Design review of the part shown in the three views and the two pictorial views. Dimensions are in mm from the part's minimum x, y and z. A direction names the side the tool comes from. Coordinates: 2 decimals unless noted, no trailing zeros. Write each loop counter-clockwise with the first axis right and the second up, starting at its lowest first coordinate (ties: lowest second). Pieces come first, ordered by that corner, then holes. Notation, with made-up numbers: (79, 19) -> (123, 19) arc R29 ccw to (123, 51) -> close; hole circle Ø9 at (1.5, -34). An arc over 180 degrees is marked (long way). Answer in a Markdown table with one row per item. Add a question column.
Item 1: Take a section at D-D, the plane y = 31. Write out the cut boundary in (x, z).
Item 2: Draft analysis for pull direction X (two halves, no side actions). For the marked faces 3 and 4, state which applies: released by +X, released by -X, zero draft, split by the parting line, or undercut.
Item 3: Take a section at B-B, the plane x = 45.5. Write out the cut boundary in (y, z).
Item 4: Clearance check with flat-ended pins moving along their axes: P1, Ø6, axis at x = 34.5, z = 41.5, coming from the +Y side; P2, Ø3.5, axis at x = 63, y = 1.5, coming from the -Z side; P3, Ø0.9, axis at x = 65.5, y = 1, coming from the +Z side; P4, Ø12, axis at x = 29, z = 6.5, coming from the -Y side. State where each tip first meets the part, or that it passes through.
Item 5: Take a section at C-C, the plane x = 63.5. Write out the cut boundary in (y, z), and give its area (3 significant figures).
Item 6: To check wall thickness, follow line 1 (X direction, y = 1, z = 24); line 2 (X direction, y = 10, z = 14.5); line 3 (Z direction, x = 63.5, y = 1.7). State the ranges of each line that lie inside material, in increasing order.
Item 7: For the marked faces 1 and 2, list the 3-axis set-ups (+Z, -Z, +X, -X, +Y, -Y) from which the entire face can be reached by the end or side of a thin tool; tool diameter is ignored.
Item 8: Take a section at A-A, the plane z = 24.25. Write out the cut boundary in (x, y).
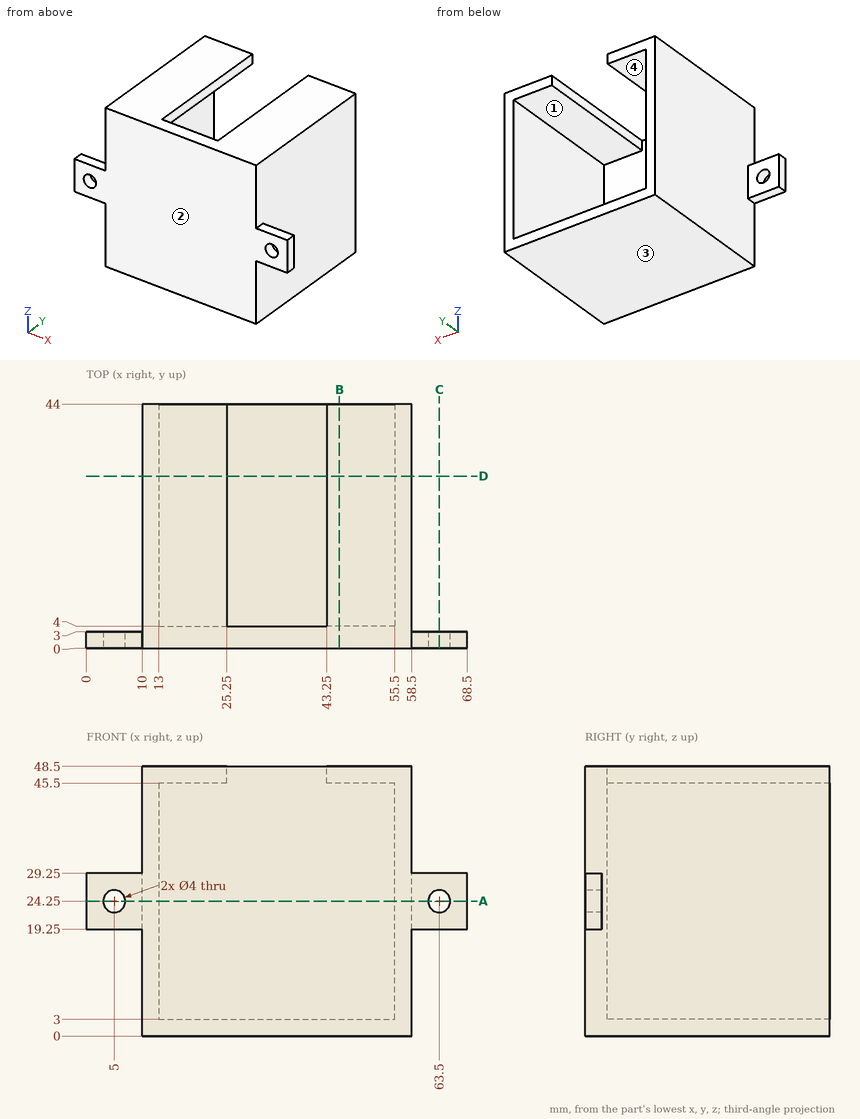
Answers:
| question | item | result |
|---|---|---|
| 1 | outline | (10, 0) -> (58.5, 0) -> (58.5, 48.5) -> (43.25, 48.5) -> (43.25, 45.5) -> (55.5, 45.5) -> (55.5, 3) -> (13, 3) -> (13, 45.5) -> (25.25, 45.5) -> (25.25, 48.5) -> (10, 48.5) -> close |
| 2 | face 3 | zero draft |
| 2 | face 4 | undercut |
| 3 | outline | (0, 0) -> (44, 0) -> (44, 3) -> (4, 3) -> (4, 45.5) -> (44, 45.5) -> (44, 48.5) -> (0, 48.5) -> close |
| 4 | P1 | stops at y = 4 |
| 4 | P2 | stops at z = 19.25 |
| 4 | P3 | stops at z = 29.25 |
| 4 | P4 | stops at y = 0 |
| 5 | outline | (0, 19.25) -> (3, 19.25) -> (3, 22.25) -> (0, 22.25) -> close; (0, 26.25) -> (3, 26.25) -> (3, 29.25) -> (0, 29.25) -> close |
| 5 | area | 18.0 mm^2 |
| 6 | line 1 | x = 0 to 3.02, 6.98 to 61.52, 65.48 to 68.5 |
| 6 | line 2 | x = 10 to 13, 55.5 to 58.5 |
| 6 | line 3 | z = 19.25 to 22.25, 26.25 to 29.25 |
| 7 | face 1 | +Y |
| 7 | face 2 | +Z, -Z, +X, -X, -Y |
| 8 | outline | (0, 0) -> (3, 0) -> (3, 3) -> (0, 3) -> close; (7, 0) -> (61.5, 0) -> (61.5, 3) -> (58.5, 3) -> (58.5, 44) -> (55.5, 44) -> (55.5, 4) -> (13, 4) -> (13, 44) -> (10, 44) -> (10, 3) -> (7, 3) -> close; (65.5, 0) -> (68.5, 0) -> (68.5, 3) -> (65.5, 3) -> close |
